Build history of the part. All positions in model axes, mm. A direction names the side the tool comes from. Round coordinates to 2 decimals unless told otherwise and drop trailing zeros. Loops run counter-clockwise (first coordinate to the right, second up) from the corner with the lowest first, then second, coordinate; pieces in that order, holes last. Notation, with made-up numbers: (9.5, 8) - (13.5, 8) arc R28 cw to (13.5, 30) - close; hole circle Ø4 at (-9, -36). An arc over 180 degrees is marked (long way). Answer as CSV lines item,"result". Start each with the question number.
```python
from build123d import *

# Parameters (mm, degrees)
SKETCH1_R           = 60
SKETCH1_R_2         = 1.35
SKETCH1_R_3         = 4
BOSS_EXTRUDE1_DEPTH = 10
CUT_EXTRUDE1_DEPTH  = 8
SKETCH6_R           = 60
SKETCH6_W           = 38.400000003
SKETCH6_H           = 51.500000005
BOSS_EXTRUDE2_DEPTH = 8
CHAMFER1_SIZE       = 5
CUT_EXTRUDE6_DEPTH  = 87.34813258
SKETCH13_W          = 159.365981606
SKETCH13_H          = 138.277350875
CUT_EXTRUDE7_DEPTH  = 6.95
SKETCH14_R          = 2.1
CUT_EXTRUDE8_DEPTH  = 86.569284793
SKETCH15_R          = 4
CUT_EXTRUDE9_DEPTH  = 7.05
SKETCH16_W          = 157.574812473
SKETCH16_H          = 128.039677695
CUT_EXTRUDE10_DEPTH = 3.05
SKETCH17_R          = 100
SKETCH17_R_2        = 50
CUT_EXTRUDE11_DEPTH = 86.229103011
SKETCH18_R          = 2.25
CUT_EXTRUDE12_DEPTH = 2.5
LPATTERN1_COUNT     = 3
LPATTERN1_PITCH     = 17
SKETCH19_R          = 2.25
CUT_EXTRUDE13_DEPTH = 2.5
SKETCH20_R          = 2.25
CUT_EXTRUDE14_DEPTH = 2.5
SKETCH21_R          = 2.25
CUT_EXTRUDE15_DEPTH = 2.5
LPATTERN2_COUNT     = 3
LPATTERN2_PITCH     = 17


with BuildPart() as part:
    # Sketch1 → Boss-Extrude1 (new body)
    with BuildSketch(Plane(origin=(0, 0, 0), x_dir=(1, 0, 0), z_dir=(0, 1, 0))):
        with Locations(Location((0, 0, 0), (0, 0, 270))):
            Circle(SKETCH1_R)
        with Locations(Location((-15, 4.5, 0), (0, 0, 270))):
            Circle(SKETCH1_R_2, mode=Mode.SUBTRACT)
        with Locations(Location((-15, -12.5, 0), (0, 0, 270))):
            Circle(SKETCH1_R_2, mode=Mode.SUBTRACT)
        with Locations(Location((-15, -29.5, 0), (0, 0, 270))):
            Circle(SKETCH1_R_2, mode=Mode.SUBTRACT)
        with Locations(Location((-8.5, -35.8, 0), (0, 0, 270))):
            Circle(SKETCH1_R_2, mode=Mode.SUBTRACT)
        with Locations(Location((8.5, -35.8, 0), (0, 0, 270))):
            Circle(SKETCH1_R_2, mode=Mode.SUBTRACT)
        with Locations(Location((15, -29.5, 0), (0, 0, 270))):
            Circle(SKETCH1_R_2, mode=Mode.SUBTRACT)
        with Locations(Location((15, -12.5, 0), (0, 0, 270))):
            Circle(SKETCH1_R_2, mode=Mode.SUBTRACT)
        with Locations(Location((15, 4.5, 0), (0, 0, 270))):
            Circle(SKETCH1_R_2, mode=Mode.SUBTRACT)
        with Locations(Location((0, 0, 0), (0, 0, 270))):
            Circle(SKETCH1_R_3, mode=Mode.SUBTRACT)
    extrude(amount=BOSS_EXTRUDE1_DEPTH)

    # Sketch2 → Cut-Extrude1 (cut)
    with BuildSketch(Plane(origin=(0, 10, 0), x_dir=(1, 0, 0), z_dir=(0, 1, 0))):
        Polygon((-12.199837774, 12.50015833), (-12.200428272, -32.999841666), (12.199571726, -33.000158329), (12.200162224, 12.499841668), align=None)
    extrude(amount=-CUT_EXTRUDE1_DEPTH, mode=Mode.SUBTRACT)

    # Sketch6 → Boss-Extrude2 (add)
    with BuildSketch(Plane(origin=(0, 10, 0), x_dir=(1, 0, 0), z_dir=(0, 1, 0))):
        with Locations(Location((0, 0, 0), (0, 0, 270))):
            Circle(SKETCH6_R)
        with Locations((0.000162221, -13.25024918)):
            Rectangle(SKETCH6_W, SKETCH6_H, mode=Mode.SUBTRACT)
    extrude(amount=BOSS_EXTRUDE2_DEPTH)

    # Chamfer1
    chamfer1_edges = [part.edges().sort_by_distance(p)[0] for p in [
        (-19.19983778, 14, -12.499750822),
        (19.200162223, 14, -12.499750822),
    ]]
    chamfer(chamfer1_edges, length=CHAMFER1_SIZE)

    # Sketch12 → Cut-Extrude6 (cut, through all)
    with BuildSketch(Plane(origin=(0, 2, 0), x_dir=(1, 0, 0), z_dir=(0, 1, 0))):
        Polygon((12.200162224, 12.499841668), (-12.199837774, 12.50015833), (-12.200428272, -32.999841666), (12.199571726, -33.000158329), align=None)
    extrude(amount=-CUT_EXTRUDE6_DEPTH, mode=Mode.SUBTRACT)

    # Sketch13 → Cut-Extrude7 (cut)
    with BuildSketch(Plane(origin=(0, 18, 0), x_dir=(1, 0, 0), z_dir=(0, 1, 0))):
        with Locations((-0.934306425, -1.920871548)):
            Rectangle(SKETCH13_W, SKETCH13_H)
    extrude(amount=-CUT_EXTRUDE7_DEPTH, mode=Mode.SUBTRACT)

    # Sketch14 → Cut-Extrude8 (cut, through all)
    with BuildSketch(Plane.XZ):
        with Locations(Location((-34.640259625, 20.004835303, 0), (0, 0, 270))):
            Circle(SKETCH14_R)
        with Locations(Location((34.63707466, 20.003132998, 0), (0, 0, 270))):
            Circle(SKETCH14_R)
        with Locations(Location((0.001, -39.995774325, 0), (0, 0, 270))):
            Circle(SKETCH14_R)
    extrude(amount=-CUT_EXTRUDE8_DEPTH, mode=Mode.SUBTRACT)

    # Sketch15 → Cut-Extrude9 (cut)
    with BuildSketch(Plane.XZ):
        with Locations(Location((34.63707466, 20.003132998, 0), (0, 0, 270))):
            Circle(SKETCH15_R)
        with Locations(Location((-34.640259625, 20.004835303, 0), (0, 0, 270))):
            Circle(SKETCH15_R)
        with Locations(Location((0.001, -39.995774325, 0), (0, 0, 270))):
            Circle(SKETCH15_R)
    extrude(amount=-CUT_EXTRUDE9_DEPTH, mode=Mode.SUBTRACT)

    # Sketch16 → Cut-Extrude10 (cut)
    with BuildSketch(Plane.XZ):
        with Locations((0.243421441, -1.785090563)):
            Rectangle(SKETCH16_W, SKETCH16_H)
    extrude(amount=-CUT_EXTRUDE10_DEPTH, mode=Mode.SUBTRACT)

    # Sketch17 → Cut-Extrude11 (cut, through all)
    with BuildSketch(Plane(origin=(0, 11.05, 0), x_dir=(1, 0, 0), z_dir=(0, 1, 0))):
        Circle(SKETCH17_R)
        with Locations(Location((0, 0, 0), (0, 0, 270))):
            Circle(SKETCH17_R_2, mode=Mode.SUBTRACT)
    extrude(amount=-CUT_EXTRUDE11_DEPTH, mode=Mode.SUBTRACT)

    # Sketch18 → Cut-Extrude12 (cut)
    with BuildSketch(Plane.XZ.offset(-3.05)):
        with Locations(Location((15, 29.5, 0), (0, 0, 270))):
            Circle(SKETCH18_R)
    cut_extrude12 = extrude(amount=-CUT_EXTRUDE12_DEPTH, mode=Mode.SUBTRACT)

    # LPattern1: Cut-Extrude12 ×3
    with Locations(*[(0, 0, -i * LPATTERN1_PITCH) for i in range(1, LPATTERN1_COUNT)]):
        add(cut_extrude12, mode=Mode.SUBTRACT)

    # Sketch19 → Cut-Extrude13 (cut)
    with BuildSketch(Plane.XZ.offset(-3.05)):
        with Locations(Location((8.5, 35.8, 0), (0, 0, 270))):
            Circle(SKETCH19_R)
    extrude(amount=-CUT_EXTRUDE13_DEPTH, mode=Mode.SUBTRACT)

    # Sketch20 → Cut-Extrude14 (cut)
    with BuildSketch(Plane.XZ.offset(-3.05)):
        with Locations(Location((-8.5, 35.8, 0), (0, 0, 270))):
            Circle(SKETCH20_R)
    extrude(amount=-CUT_EXTRUDE14_DEPTH, mode=Mode.SUBTRACT)

    # Sketch21 → Cut-Extrude15 (cut)
    with BuildSketch(Plane.XZ.offset(-3.05)):
        with Locations(Location((-15, 29.5, 0), (0, 0, 270))):
            Circle(SKETCH21_R)
    cut_extrude15 = extrude(amount=-CUT_EXTRUDE15_DEPTH, mode=Mode.SUBTRACT)

    # LPattern2: Cut-Extrude15 ×3
    with Locations(*[(0, 0, -i * LPATTERN2_PITCH) for i in range(1, LPATTERN2_COUNT)]):
        add(cut_extrude15, mode=Mode.SUBTRACT)


solid = part.part
```
Q1. Band-saw the part on D-D, the plane z = 43.5. List the corners of the cut face in (x, y), then the cut area to 3 significant figures.
Q2. Band-saw the part on C-C, the plane z = -33.5. List the corners of the cut face in (x, y).
Q3. Band-saw the part on A-A, the plane z = -4.5. List the corners of the cut face in (x, y).
Q4. Two-plate mould, pull along Z, no slides. Class faces 4 (the flat face through (-1, 3.05, -22)), 5 (the cylindrical face through (-16.369, 4.282, 14.286)): released by +Z, released by -Z, zero draft, split by the parting line, or undercut.
Q5. Band-saw the part on B-B, the plane x = -8.5. Give the number of separate pieces and of enclosed holes in the cut face, then the cut area to 3 significant figures.
Q6. Tool access for faces 1 (the flat face through (13.5, 5.55, 29.5)), 2 (the flat face through (13, 10, 19)), 3 (the cylindrical face through (8.56, 7.74, 34.45)): list every direction of +Z, -Z, +X, -X, +Y, -Y with a clear straight run to the whole face (end or side of a thin tool).
Q7. Pin check, flat tips, straight feed: pin 1 Ø3 at (y, z) = (5, -24.5) entering from -X; pin 2 Ø4 at (x, y) = (26.5, 10) entering from +Z; pin 3 Ø0.8 at (y, z) = (10.5, 11) entering from -X; pin 4 Ø3.5 at (x, z) = (9.5, 34.5) entering from -Y. Stop position of each tip, or through.
Q8. Wall check: probe 1 along Z at (x, y) = (3.5, 4.25); probe 2 along X at (y, z) = (8, -0.5); probe 3 along X at (y, z) = (3.75, 37). Give the ranges that are in metal, low to high. Write a range as [from, to].
Reported:
1,outline,"(-24.65, 3.05) - (24.65, 3.05) - (24.65, 11.05) - (-24.65, 11.05) - close"
1,area,"394 mm2"
2,outline,"(-37.12, 3.05) - (37.12, 3.05) - (37.12, 11.05) - (-37.12, 11.05) - close"
3,outline,"(-49.8, 3.05) - (-17.25, 3.05) - (-17.25, 5.55) - (-16.35, 5.55) - (-16.35, 10) - (-19.2, 10) - (-19.2, 11.05) - (-49.8, 11.05) - close; (-13.65, 5.55) - (-12.75, 5.55) - (-12.75, 3.05) - (-12.2, 3.05) - (-12.2, 10) - (-13.65, 10) - close; (12.2, 3.05) - (12.75, 3.05) - (12.75, 5.55) - (13.65, 5.55) - (13.65, 10) - (12.2, 10) - close; (16.35, 5.55) - (17.25, 5.55) - (17.25, 3.05) - (49.8, 3.05) - (49.8, 11.05) - (19.2, 11.05) - (19.2, 10) - (16.35, 10) - close"
4,face 4,"zero draft"
4,face 5,"undercut"
5,separate pieces,"3"
5,enclosed holes,"0"
5,area,"395 mm2"
6,face 1,"-Y"
6,face 2,"+Y"
6,face 3,"+Y, -Y"
7,pin 1,"stops at x = -44.4"
7,pin 2,"stops at z = 43.59"
7,pin 3,"stops at x = -48.86"
7,pin 4,"stops at y = 3.05"
8,probe 1,"z = [-49.88, -41.93], [-38.06, -12.5], [33, 49.88]"
8,probe 2,"x = [-50, -12.2], [12.2, 50]"
8,probe 3,"x = [-33.63, -10.4], [-6.6, 6.6], [10.4, 33.63]"
